Verification items for the finished model (mm, model axes). Face numbers are marked on the shaded views. A direction names the side the tool comes from. Coordinates: 2 decimals unless noted, no trailing zeros. Loops run counter-clockwise (first coordinate to the right, second up) from the corner with the lowest first, then second, coordinate; pieces in that order, holes last. Notation, with made-up numbers: (21.5, -20) -> (68.5, -20) arc R24 cw to (68.5, -5) -> close; hole circle Ø10 at (-22, 0). An arc over 180 degrees is marked (long way). Write item = value, one per line.
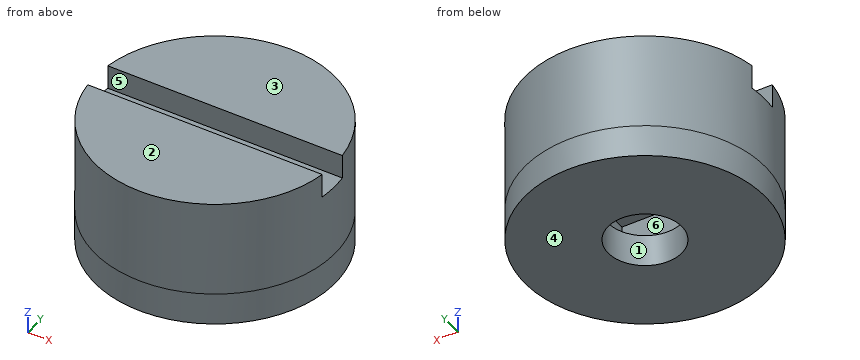
```python
from build123d import *

# Parameters (mm, degrees)
SKETCH_R        = 7.5
SKETCH_R_2      = 2.3
PAD_DEPTH       = 2
SKETCH001_R     = 7.5
PAD001_DEPTH    = 6
SKETCH002_W     = 8
SKETCH002_H     = 8
POCKET_DEPTH    = 3
SKETCH003_W     = 26.953154
SKETCH003_H     = 2
POCKET001_DEPTH = 3.5


with BuildPart() as part:
    # Sketch → Pad (new body)
    with BuildSketch(Plane.XY):
        Circle(SKETCH_R)
        Circle(SKETCH_R_2, mode=Mode.SUBTRACT)
    extrude(amount=-PAD_DEPTH)

    # Sketch001 → Pad001 (join)
    with BuildSketch(Plane.XY):
        Circle(SKETCH001_R)
    extrude(amount=PAD001_DEPTH)

    # Sketch002 → Pocket (cut)
    with BuildSketch(Plane.XY):
        Rectangle(SKETCH002_W, SKETCH002_H)
    extrude(amount=POCKET_DEPTH, mode=Mode.SUBTRACT)

    # Sketch003 (on DatumPlane) → Pocket001 (cut, symmetric)
    with BuildSketch(Plane.XY.offset(8)):
        Rectangle(SKETCH003_W, SKETCH003_H)
    extrude(amount=POCKET001_DEPTH, both=True, mode=Mode.SUBTRACT)


solid = part.part
```
1) Release check for a two-part mould opening along Z. For the marked faces 3, 4, 5 and 6 record: pulls with the +Z half, pulls with the -Z half, needs draft (parallel to the pull), parting line crosses it, or undercut.
Ans:
face_3 = pulls with the +Z half
face_4 = pulls with the -Z half
face_5 = needs draft
face_6 = undercut
2) Sectioned sample at D-D, the plane y = 0. Record the cut outline in (x, z), plus the area to 3 significant figures.
Ans:
outline = (-7.5, -2) -> (-2.3, -2) -> (-2.3, 0) -> (-4, 0) -> (-4, 3) -> (4, 3) -> (4, 0) -> (2.3, 0) -> (2.3, -2) -> (7.5, -2) -> (7.5, 4.5) -> (-7.5, 4.5) -> close
area = 64.3 mm2
3) Sectioned sample at A-A, the plane y = -3. Record the cut outline in (x, z), plus the area to 3 significant figures.
Ans:
outline = (-6.87, -2) -> (6.87, -2) -> (6.87, 6) -> (-6.87, 6) -> close; hole (-4, 0) -> (4, 0) -> (4, 3) -> (-4, 3) -> close
area = 86.0 mm2
4) Tool access check on the marked faces 1 and 2. Record the directions out of +Z, -Z, +X, -X, +Y, -Y that give a thin tool (end or side, any length) a straight path to the whole face; none if there is none.
Ans:
face_1 = -Z
face_2 = +Z, +X, -X, +Y, -Y
5) Sectioned sample at C-C, the plane z = 2.75. Record the cut outline in (x, y).
Ans:
outline = circle Ø15 at (0, 0); hole (-4, -4) -> (4, -4) -> (4, 4) -> (-4, 4) -> close
6) Depth check by flat-ended pin: pin 1 Ø1.2 at (x, z) = (-3.5, 5) entering from +Y; pin 2 Ø2.5 at (x, z) = (-2, 2) entering from -Y; pin 3 Ø3 at (x, z) = (-5.5, 2) entering from -Y. Enter the tip coordinate at first touch or a pass-through.
Ans:
pin_1 = 6.92
pin_2 = -7.46
pin_3 = -6.34
7) Material ranges on line 1 (Z direction, x = -3.25, y = -3.5); line 2 (Y direction, x = 0, z = -0.35); line 3 (Z direction, x = 2.5, y = 0), recorded low to high.
Ans:
line_1 = -2 to 0, 3 to 6
line_2 = -7.5 to -2.3, 2.3 to 7.5
line_3 = -2 to 0, 3 to 4.5
8) Sectioned sample at B-B, the plane x = 0. Record the cut outline in (y, z), plus the area to 3 significant figures.
Ans:
outline = (-7.5, -2) -> (-2.3, -2) -> (-2.3, 0) -> (-4, 0) -> (-4, 3) -> (4, 3) -> (4, 0) -> (2.3, 0) -> (2.3, -2) -> (7.5, -2) -> (7.5, 6) -> (1, 6) -> (1, 4.5) -> (-1, 4.5) -> (-1, 6) -> (-7.5, 6) -> close
area = 83.8 mm2
